from build123d import *

# Parameters (mm, degrees)
F0_R     = 7.5
F1_DEPTH = 10
F3_COUNT = 16
F3_ANGLE = 337.5
F4_R     = 2.0024063546
F5_DEPTH = 10


with BuildPart() as f1:
    # F0 (on Top) → F1 (new body)
    with BuildSketch(Plane.XY):
        with BuildLine():
            ThreePointArc((-3.6476693986, 17.115621752), (-11.0094456156, -13.6030183135), (17.5, 0))
            ThreePointArc((17.5, 0), (12.4584016864, 12.2897610807), (0.2384882949, 17.4983748769))
            ThreePointArc((0.2384882949, 17.4983748769), (-1.7152999558, 17.4157327168), (-3.6476693986, 17.115621752))
        make_face()
        Circle(F0_R, mode=Mode.SUBTRACT)
        with BuildLine():
            ThreePointArc((-3.6476693986, 17.115621752), (-1.7152999558, 17.4157327168), (0.2384882949, 17.4983748769))
            ThreePointArc((0.2384882949, 17.4983748769), (-0.1063528579, 20.2679092651), (-1.8819552556, 22.4211561793))
            ThreePointArc((-1.8819552556, 22.4211561793), (-2.2053856574, 22.3916563501), (-2.528356566, 22.3574912071))
            ThreePointArc((-2.528356566, 22.3574912071), (-3.8497636276, 19.8992154851), (-3.6476693986, 17.115621752))
        make_face()
    extrude(amount=F1_DEPTH)

    # F3: F1 ×16 about axis
    f3_axis = Axis((0, 0, 13.1933512166), (0, 0, 1))


with BuildPart() as f1_1:
    add(f1.part)
    for i in range(1, F3_COUNT):
        add(f1.part.rotate(f3_axis, i * F3_ANGLE / (F3_COUNT - 1)))

    # F4 (on face) → F5 (cut)
    with BuildSketch(Plane.XY.offset(10)):
        with Locations((-12.467992492, 0)):
            Circle(F4_R)
    extrude(amount=-F5_DEPTH, mode=Mode.SUBTRACT)


solid = f1_1.part
Verification items for the finished model (mm, model axes). A direction names the side the tool comes from. Round coordinates to 2 decimals unless told otherwise and drop trailing zeros. Loops run counter-clockwise (first coordinate to the right, second up) from the corner with the lowest first, then second, coordinate; pieces in that order, holes last. Notation, with made-up numbers: M -7.5,47.25 L 7.5,47.25 A22 cw 7.5,75.25 Z; hole C 50.5,10.5 d2. An arc over 180 degrees is marked long. Write each question's results on one line, items separated by ' | '.
1) Scan lines: L1, parallel to Y at x = -13.5, z = 2.75; L2, parallel to Y at x = -13, z = 6.75; L3, parallel to X at y = 18, z = 2.25. Record each from-to range of solid material in increasing order. Write a range as from..to.
Checks:
L1: y = -17.56..-13.11, -11.14..-1.72, 1.72..13.78 | L2: y = -17.48..-12.58, -11.72..-1.93, 1.93..13.41 | L3: x = -11.25..-7.27, -3.89..0.29, 3.27..7.61
2) Access from +Z, -Z, +X, -X, +Y, -Y to the whole of each face (thin tool, end or side, straight path). Record for faces 1 (the cylindrical face through (-11.382, -16.814, 4.93)), 2 (the cylindrical face through (8.268, 15.424, 4.93)).
Checks:
face 1: +Z, -Z, -Y | face 2: +Z, -Z
3) Section check A-A on x = -19. Record the boundary of the cut face in (y, z).
Checks:
outline: M -11.11,0 L -8.21,0 L -8.21,10 L -11.11,10 Z; M -3.96,0 L 0.25,0 L 0.25,10 L -3.96,10 Z; M 3.58,0 L 7.65,0 L 7.65,10 L 3.58,10 Z
4) Gauge pin test, flat ends, axial feed: P1, Ø1, axis at y = 8.5, z = 4, coming from the -X side; P2, Ø3, axis at x = -7, z = 4.5, coming from the -Y side; P3, Ø4, axis at y = -6, z = 6, coming from the +X side. Record the tip position at first contact, or that the pin passes through.
Checks:
P1: stops at x = -15.56 | P2: stops at y = -21.62 | P3: stops at x = 21.62
5) Section check B-B on z = 4.5. State how many separate pieces and enclosed holes the cut face has, then the cut area to 3 significant figures.
Checks:
separate pieces: 1 | enclosed holes: 2 | area: 1,040 mm2
